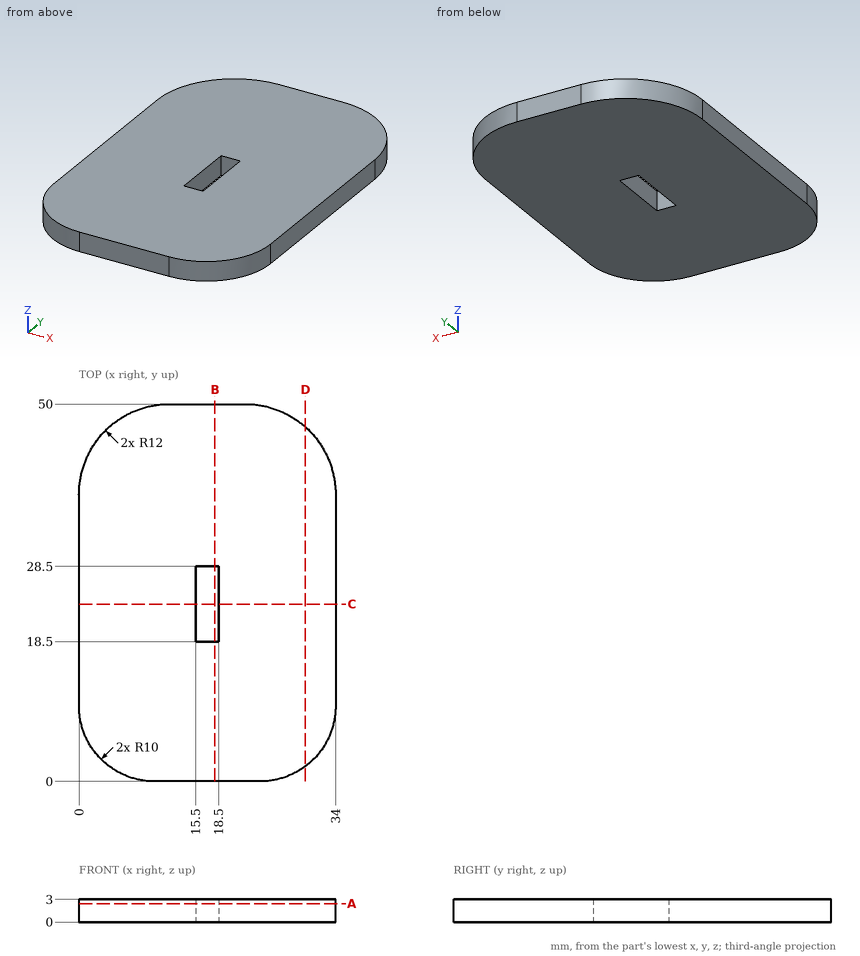
The drawing under review shows one solid part. Ordinate dimensions are in mm from its lowest x, y, z. Coordinates: 2 decimals unless noted, no trailing zeros. Loops run counter-clockwise (first coordinate to the right, second up) from the corner with the lowest first, then second, coordinate; pieces in that order, holes last.
Item 1: Wall thickness on L1, parallel to X at y = 28, z = 0.2; L2, parallel to Y at x = 16.5, z = 1.1; L3, parallel to Y at x = 11.5, z = 2.55: over which ranges is each line inside the solid? List them lowest first.
Completed:
L1: x = 0 to 15.5, 18.5 to 34
L2: y = 0 to 18.5, 28.5 to 50
L3: y = 0 to 49.99
Item 2: Add section D-D (x = 30). Write out the cut boundary in (y, z).
Completed:
outline: (2, 0) - (46.94, 0) - (46.94, 3) - (2, 3) - close
Item 3: Clearance check with flat-ended pins moving along their axes: pin 1 (12 mm diameter, centred on x = 21.5, y = 24.5, fed in from -Z); pin 2 (1 mm diameter, centred on y = 7.5, z = 0.5, fed in from +X). State where each tip first meets the part, or that it passes through.
Completed:
pin 1: stops at z = 0
pin 2: stops at x = 33.8
Item 4: Add section B-B (x = 18). Write out the cut boundary in (y, z).
Completed:
outline: (0, 0) - (18.5, 0) - (18.5, 3) - (0, 3) - close; (28.5, 0) - (50, 0) - (50, 3) - (28.5, 3) - close
Item 5: Add section A-A (z = 2.45). Write out the cut boundary in (x, y).
Completed:
outline: (0, 10) arc R10 ccw to (10, 0) - (24, 0) arc R10 ccw to (34, 10) - (34, 38) arc R12 ccw to (22, 50) - (12, 50) arc R12 ccw to (0, 38) - close; hole (15.5, 18.5) - (18.5, 18.5) - (18.5, 28.5) - (15.5, 28.5) - close
Item 6: Add section C-C (y = 23.5). Write out the cut boundary in (x, z), and give its area (3 significant figures).
Completed:
outline: (0, 0) - (15.5, 0) - (15.5, 3) - (0, 3) - close; (18.5, 0) - (34, 0) - (34, 3) - (18.5, 3) - close
area: 93.0 mm2
